Verification items for the finished model (mm, model axes). Face numbers are marked on the shaded views. A direction names the side the tool comes from. Round coordinates to 2 decimals unless told otherwise and drop trailing zeros. Order: outer loops, then holes, each group sorted by start corner. A loop starts at its lowest first (then second) coordinate and runs counter-clockwise, first axis right, second up. Notation, with made-up numbers: M 17,27.5 L 24,27.5 A22 cw 24,51.5 Z; hole C 55,-35 d7. An arc over 180 degrees is marked long. Use one line per item in the form item = value. Start each with the question number.
Item 1: Cross-section at C-C on z = -59. Enter the section's corners in (x, y).
Item 2: Cross-section at B-B on y = 50. Enter the section's corners in (x, z).
Item 3: Tool access check on the marked faces 1 and 2. Record the directions out of +Z, -Z, +X, -X, +Y, -Y that give a thin tool (end or side, any length) a straight path to the whole face; none if there is none.
Item 4: Go/stop test with flat-tipped pins: pin 1 Ø7.5 at (x, y) = (673.1, 38.1) entering from -Z; pin 2 Ø6 at (x, z) = (609.6, -44.45) entering from +Y; pin 3 Ø1.5 at (x, z) = (570.5, -55.5) entering from +Y. Record where each tip stops, or that it passes through.
Item 5: Cross-section at A-A on x = 706.5. Enter the section's corners in (y, z), then the cut area to 3 significant figures.
Item 6: Thickness scan on probe 1 along Z at (x, y) = (355, 5); probe 2 along Z at (x, y) = (376.5, 66.5); probe 3 along Y at (x, z) = (197.5, -72). Record the ranges inside material, lowest first. Write a range as [from, to].
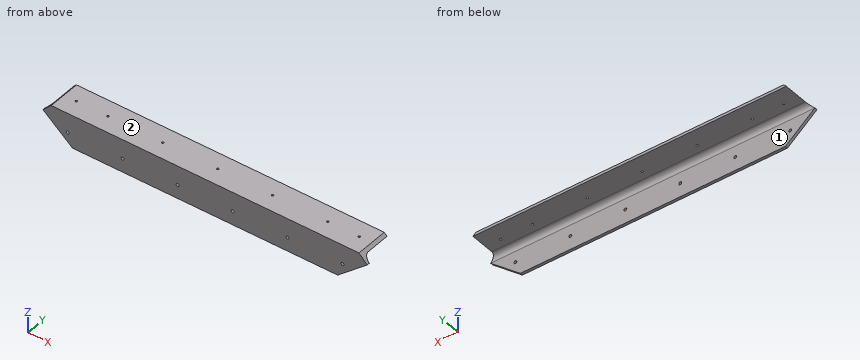
from build123d import *

# Parameters (mm, degrees)
BOSS_EXTRUDE1_DEPTH              = 838.2
FILLET1_R                        = 12.7
F_17_64_0_26563_DIAMETER_HOLE1_D = 6.747002
LPATTERN1_COUNT                  = 6
LPATTERN1_PITCH                  = 127
CUT_EXTRUDE3_DEPTH               = 846.098881788
CUT_EXTRUDE4_DEPTH               = 846.098881788
CUT_EXTRUDE5_DEPTH               = 845.55
CUT_EXTRUDE6_DEPTH               = 845.55
F_3_16_0_1875_DIAMETER_HOLE1_D   = 4.7625
LPATTERN2_COUNT                  = 3
LPATTERN2_PITCH                  = 127
LPATTERN3_COUNT                  = 3
LPATTERN3_PITCH                  = 127
F_3_16_0_1875_DIAMETER_HOLE3_D   = 4.7625


with BuildPart() as part:
    # Sketch1 → Boss-Extrude1 (new body)
    with BuildSketch(Plane(origin=(0, 0, 0), x_dir=(0, 0, -1), z_dir=(1, 0, 0))):
        Polygon((0, 0), (76.2, 0), (76.2, 6.35), (6.35, 6.35), (6.35, 76.2), (0, 76.2), align=None)
    extrude(amount=BOSS_EXTRUDE1_DEPTH)

    # Fillet1
    fillet1_edges = [part.edges().sort_by_distance(p)[0] for p in [
        (419.1, 6.35, -6.35),
    ]]
    fillet(fillet1_edges, radius=FILLET1_R)

    # 17/64 (0.26563) Diameter Hole1 (through all)
    with Locations(Plane(origin=(0, 6.35, 0), x_dir=(1, 0, 0), z_dir=(0, 1, 0))):
        with Locations((101.6, 44.45)):
            f_17_64_0_26563_diameter_hole1 = Hole(F_17_64_0_26563_DIAMETER_HOLE1_D / 2)

    # LPattern1: 17/64 (0.26563) Diameter Hole1 ×6
    with Locations(*[(i * LPATTERN1_PITCH, 0, 0) for i in range(1, LPATTERN1_COUNT)]):
        add(f_17_64_0_26563_diameter_hole1, mode=Mode.SUBTRACT)

    # Sketch7 → Cut-Extrude3 (cut, through all)
    with BuildSketch(Plane.XZ):
        Polygon((63.5, 0), (-28.052450059, 0), (-28.052450059, -91.552450059), align=None)
    extrude(amount=-CUT_EXTRUDE3_DEPTH, mode=Mode.SUBTRACT)

    # Sketch8 → Cut-Extrude4 (cut, through all)
    with BuildSketch(Plane.XZ):
        Polygon((774.7, 0), (864.325160155, 0), (864.325160155, -89.625160155), align=None)
    extrude(amount=-CUT_EXTRUDE4_DEPTH, mode=Mode.SUBTRACT)

    # Sketch12 → Cut-Extrude5 (cut, through all)
    with BuildSketch(Plane(origin=(0, 6.35, 0), x_dir=(1, 0, 0), z_dir=(0, 1, 0))):
        Polygon((44.549132772, 18.950867228), (112.775992426, 76.2), (-12.7, 76.2), align=None)
    extrude(amount=-CUT_EXTRUDE5_DEPTH, mode=Mode.SUBTRACT)

    # Sketch14 → Cut-Extrude6 (cut, through all)
    with BuildSketch(Plane(origin=(0, 6.35, 0), x_dir=(1, 0, 0), z_dir=(0, 1, 0))):
        Polygon((793.650867228, 18.950867228), (850.9, 76.2), (725.424007574, 76.2), align=None)
    extrude(amount=-CUT_EXTRUDE6_DEPTH, mode=Mode.SUBTRACT)

    # 3/16 (0.1875) Diameter Hole1 (through all)
    with Locations(Plane(origin=(0, 0, -6.35), x_dir=(-1, 0, 0), z_dir=(0, 0, -1))):
        with Locations((-419.1, 38.1)):
            f_3_16_0_1875_diameter_hole1 = Hole(F_3_16_0_1875_DIAMETER_HOLE1_D / 2)

    # LPattern2: 3/16 (0.1875) Diameter Hole1 ×3
    with Locations(*[(-i * LPATTERN2_PITCH, 0, 0) for i in range(1, LPATTERN2_COUNT)]):
        add(f_3_16_0_1875_diameter_hole1, mode=Mode.SUBTRACT)

    # LPattern3: 3/16 (0.1875) Diameter Hole1 ×3
    with Locations(*[(i * LPATTERN3_PITCH, 0, 0) for i in range(1, LPATTERN3_COUNT)]):
        add(f_3_16_0_1875_diameter_hole1, mode=Mode.SUBTRACT)

    # 3/16 (0.1875) Diameter Hole3 (through all)
    with Locations(Plane(origin=(0, 0, -6.35), x_dir=(-1, 0, 0), z_dir=(0, 0, -1))):
        with Locations((-746.125, 38.1), (-92.075, 38.1)):
            Hole(F_3_16_0_1875_DIAMETER_HOLE3_D / 2)


solid = part.part
Output values:
q1.outline = M 92.28,0 L 745.92,0 L 745.92,6.35 L 92.28,6.35 Z
q2.outline = M 57.15,-6.35 L 781.05,-6.35 L 774.7,0 L 63.5,0 Z
q3.face_1 = -Z, +X, -X, +Y
q3.face_2 = +Z, +X, -X, +Y, -Y
q4.pin_1 = -6.35
q4.pin_2 = through
q4.pin_3 = 6.35
q5.outline = M 0,-76.2 L 6.35,-76.2 L 6.35,-19.05 A12.7 cw 19.05,-6.35 L 76.2,-6.35 L 76.2,0 L 0,0 Z
q5.area = 962 mm2
q6.probe_1 = [-76.2, -47.77], [-41.13, 0]
q6.probe_2 = [-6.35, 0]
q6.probe_3 = [0, 6.35]
